from build123d import *

# Parameters (mm, degrees)
SKETCH1_R           = 4
BOSS_EXTRUDE2_DEPTH = 3


with BuildPart() as part:
    # Sketch1 → Boss-Extrude2 (new body)
    with BuildSketch(Plane.XY):
        Polygon((160.82, 34.005), (195.645, 34.005), (198.82, 34.005), (198.82, 37.18), (198.82, 72.005), (232.325, 72.005), (232.325, 325.985), (198.82, 325.985), (198.82, 360.81), (198.82, 363.985), (195.645, 363.985), (160.82, 363.985), (160.82, 397.99), (34.825, 397.99), (34.825, 363.985), (0, 363.985), (-3.175, 363.985), (-3.175, 266.995), (12.005, 266.995), (12.005, 252), (12.005, 217.17), (46.835, 217.17), (46.835, 213.995), (76.83, 213.995), (76.83, 183.995), (46.835, 183.995), (46.835, 180.82), (12.005, 180.82), (12.005, 145.99), (12.005, 130.995), (-3.175, 130.995), (-3.175, 34.005), (0, 34.005), (34.825, 34.005), (34.825, 0), (160.82, 0), align=None)
        with Locations((60, 19.005)):
            Circle(SKETCH1_R, mode=Mode.SUBTRACT)
        with Locations((135.645, 19.005)):
            Circle(SKETCH1_R, mode=Mode.SUBTRACT)
        with Locations((213.82, 97.18)):
            Circle(SKETCH1_R, mode=Mode.SUBTRACT)
        with Locations((60, 378.985)):
            Circle(SKETCH1_R, mode=Mode.SUBTRACT)
        with Locations((135.645, 378.985)):
            Circle(SKETCH1_R, mode=Mode.SUBTRACT)
        with Locations((213.82, 300.81)):
            Circle(SKETCH1_R, mode=Mode.SUBTRACT)
    extrude(amount=BOSS_EXTRUDE2_DEPTH)


solid = part.part
Could you check a few things on this model? Use its own coordinates, in mm. Give positions to 0.01 mm unless a question says otherwise; leave off trailing zeros. Order: outer loops, then holes, each group sorted by start corner. A loop starts at its lowest first (then second) coordinate and runs counter-clockwise, first axis right, second up. Notation, with made-up numbers: (47, 82.25) - (101, 82.25) arc R22 ccw to (101, 99.25) - close; hole circle Ø5 at (37, -1.75). An arc over 180 degrees is marked (long way). One line per question, with ' | ' between items. Start each with the question number.
Item 1: I want a section at C-C on y = 97.18. Write out the boundary of the cut face in (x, z) (3 decimals).
Item 2: Thinking about a two-plate mould opening in Y: for faces 1 (the flat face through (113, 202, 0)), 2 (the cylindrical face through (63.815, 20.206, 1.479)), which applies, pulls with the +Y half, pulls with the -Y half, needs draft (parallel to the pull), parting line crosses it, or undercut?
Item 3: I need wall thicknesses on probe 1 along Y at (x, z) = (60, 1.5) (3 decimals); probe 2 along Y at (x, z) = (213.82, 1.5) (3 decimals); probe 3 along Y at (x, z) = (49, 1) (3 decimals). Which ranges of each line are inside material? Lowest first, please. Write a range as [from, to].
Item 4: I want a section at D-D on x = 24.5. Write out the boundary of the cut face in (y, z) (3 decimals).
Item 5: I want a section at A-A on x = 60. Write out the boundary of the cut face in (y, z) (3 decimals), then the cut area to 3 significant figures.
Item 6: I want a section at B-B on x = 213.82. Write out the boundary of the cut face in (y, z) (3 decimals).
Item 7: I'm going to push flat-ended pins straight in: pin 1 Ø13 at (x, y) = (60, 378.985) entering from +Z; pin 2 Ø1.5 at (x, z) = (171, 1.5) entering from -Y (3 decimals); pin 3 Ø1.5 at (y, z) = (182.5, 1.5) entering from -X (3 decimals). Where does each tip first touch, or does it pass through?
Verdict:
1) outline: (-3.175, 0) - (209.82, 0) - (209.82, 3) - (-3.175, 3) - close; (217.82, 0) - (232.325, 0) - (232.325, 3) - (217.82, 3) - close
2) face 1: needs draft | face 2: undercut
3) probe 1: [0, 15.005], [23.005, 183.995], [213.995, 374.985], [382.985, 397.99] | probe 2: [72.005, 93.18], [101.18, 296.81], [304.81, 325.985] | probe 3: [0, 183.995], [213.995, 397.99]
4) outline: (34.005, 0) - (180.82, 0) - (180.82, 3) - (34.005, 3) - close; (217.17, 0) - (363.985, 0) - (363.985, 3) - (217.17, 3) - close
5) outline: (0, 0) - (15.005, 0) - (15.005, 3) - (0, 3) - close; (23.005, 0) - (183.995, 0) - (183.995, 3) - (23.005, 3) - close; (213.995, 0) - (374.985, 0) - (374.985, 3) - (213.995, 3) - close; (382.985, 0) - (397.99, 0) - (397.99, 3) - (382.985, 3) - close | area: 1,060 mm^2
6) outline: (72.005, 0) - (93.18, 0) - (93.18, 3) - (72.005, 3) - close; (101.18, 0) - (296.81, 0) - (296.81, 3) - (101.18, 3) - close; (304.81, 0) - (325.985, 0) - (325.985, 3) - (304.81, 3) - close
7) pin 1: z = 3 | pin 2: y = 34.005 | pin 3: x = 46.835
